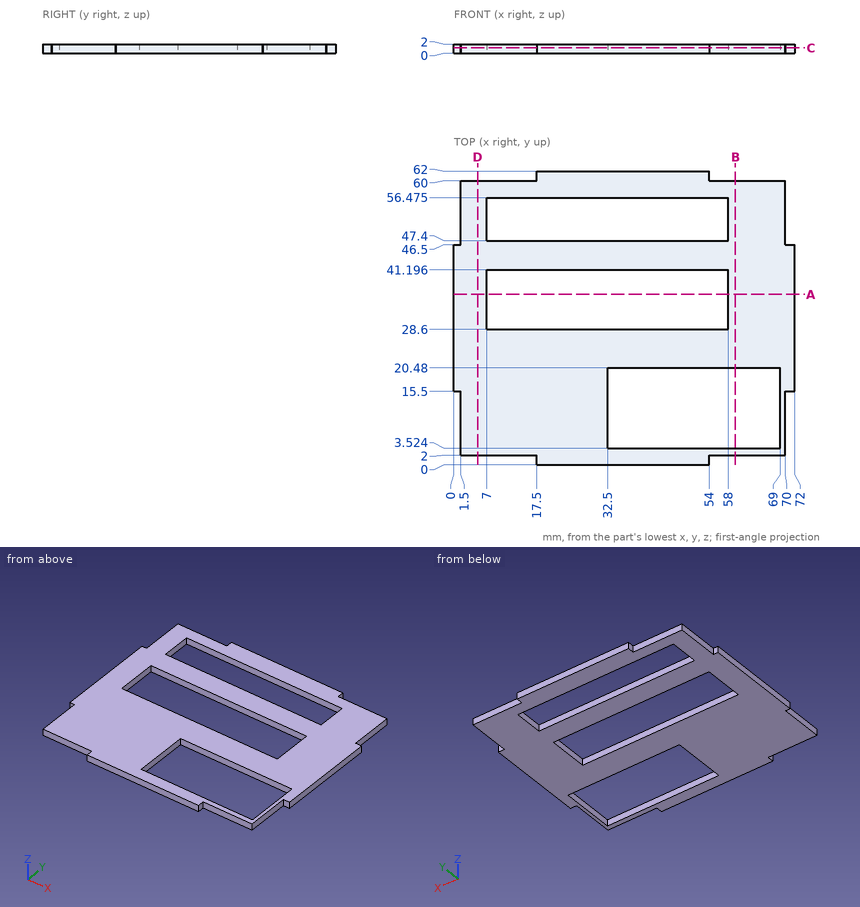
Print and shaded views of the part. All mm, measured from the part's lowest x, y and z. Coordinates: 2 decimals unless noted, no trailing zeros. Loops run counter-clockwise (first coordinate to the right, second up) from the corner with the lowest first, then second, coordinate; pieces in that order, holes last. Notation, with made-up numbers: (-35, 57.5) -> (23, 57.5) arc R12 ccw to (23, 63.5) -> close; hole circle Ø1 at (4, 75). An arc over 180 degrees is marked (long way). Use one line per item in the form item = value. Start each with the question number.
(1) Probe probe 1 along Y at (x, z) = (28.5, 0.5) (1 decimal); probe 2 along Y at (x, z) = (51, 0.7) (1 decimal); probe 3 along Y at (x, z) = (13, 1.55) (1 decimal). List the from-to ranges inside material, lowest first. Write a range as from..to.
(2) Cut at D-D on x = 5. Give the cut face in (y, z), and give its area (3 significant figures).
(3) Cut at A-A on y = 36. Give the cut face in (x, z).
(4) Cut at B-B on x = 59.5. Give the cut face in (y, z).
(5) Flat gauge pins, fed straight in: pin 1 (0.6 mm diameter, centred on y = 11, z = 1, fed in from +X); pin 2 (0.6 mm diameter, centred on y = 51, z = 1, fed in from -X); pin 3 (1.2 mm diameter, centred on x = 0.5, z = 0.5, fed in from -Y). Where does each tip first touch, or does it go through?
(6) Cut at C-C on z = 1.2. Give the number of separate pieces and of enclosed holes in the cut face, and give its area (3 significant figures).
Values:
q1.probe_1 = 0..28.6, 41.2..47.4, 56.5..62
q1.probe_2 = 0..3.5, 20.5..28.6, 41.2..47.4, 56.5..62
q1.probe_3 = 2..28.6, 41.2..47.4, 56.5..60
q2.outline = (2, 0) -> (60, 0) -> (60, 2) -> (2, 2) -> close
q2.area = 116 mm2
q3.outline = (0, 0) -> (7, 0) -> (7, 2) -> (0, 2) -> close; (58, 0) -> (72, 0) -> (72, 2) -> (58, 2) -> close
q4.outline = (2, 0) -> (3.52, 0) -> (3.52, 2) -> (2, 2) -> close; (20.48, 0) -> (60, 0) -> (60, 2) -> (20.48, 2) -> close
q5.pin_1 = 70
q5.pin_2 = 1.5
q5.pin_3 = 15.5
q6.separate_pieces = 1
q6.enclosed_holes = 3
q6.area = 2,500 mm2
